The listing builds one solid part. Answer for the finished solid, in the listing's coordinates (mm). A direction names the side the tool comes from. Round coordinates to 2 decimals unless told otherwise and drop trailing zeros. One line per item, written item: value. Start each with the question number.
(1) For a pull along Y with two mould halves and no side action, classify faces 3 (the flat face through (8, 1, 0)), 4 (the flat face through (-3.12, 5.5, 8.59)), 5 (the cylindrical face through (-4.88, 37.18, 26.75)) as released by +Y, released by -Y, zero draft, split by the parting line, or undercut.
(2) Consider probe 1 along Y at (x, z) = (0, 1); probe 2 along Z at (x, y) = (13, -11); probe 3 along Y at (x, z) = (5, 10.25). Determine where each line is inside the solid, lowest interval first.
(3) For faces 1 (the flat face through (3.21, 5.45, 8.59)), 2 (the cylindrical face through (-4.88, 37.18, 0.25)), determine the directions among +Z, -Z, +X, -X, +Y, -Y from which every point of the face is accessible in a straight line to the end or side of a thin tool.
(4) Given P1, Ø8, axis at x = -26.5, z = 13.5, coming from the +Y side; P2, Ø2, axis at y = 1.5, z = 7.5, coming from the -X side; P3, Ø12, axis at x = -0.5, z = 13, coming from the +Y side, each flat-ended and moving along its own axis, determine where each tip first touches the part or whether it passes through.
```python
from build123d import *

# Parameters (mm, degrees)
ESQUISSE1_R             = 37.5
ESQUISSE1_R_2           = 2.15
BOSS_EXTRU_1_DEPTH      = 15
ESQUISSE2_R             = 37.5
ESQUISSE2_R_2           = 18.85
BOSS_EXTRU_2_DEPTH      = 12
ENL_V_MAT_EXTRU_9_DEPTH = 13
CHANFREIN1_SIZE         = 1


with BuildPart() as part:
    # Esquisse1 → Boss.-Extru.1 (new body)
    with BuildSketch(Plane.XY):
        Circle(ESQUISSE1_R)
        Circle(ESQUISSE1_R_2, mode=Mode.SUBTRACT)
    extrude(amount=BOSS_EXTRU_1_DEPTH)

    # Esquisse2 → Boss.-Extru.2 (add)
    with BuildSketch(Plane.XY.offset(15)):
        Circle(ESQUISSE2_R)
        Circle(ESQUISSE2_R_2, mode=Mode.SUBTRACT)
    extrude(amount=BOSS_EXTRU_2_DEPTH)

    # Esquisse9 → Enlèv. mat.-Extru.9 (cut)
    with BuildSketch(Plane.XY.offset(15)):
        Polygon((6.325, -3.651740453), (6.325, 3.651740453), (0, 7.303480905), (-6.325, 3.651740453), (-6.325, -3.651740453), (0, -7.303480905), align=None)
    extrude(amount=-ENL_V_MAT_EXTRU_9_DEPTH, mode=Mode.SUBTRACT)

    # Chanfrein1
    chanfrein1_edges = [part.edges().sort_by_distance(p)[0] for p in [
        (-18.85, 0, 27),
    ]]
    chamfer(chanfrein1_edges, length=CHANFREIN1_SIZE)

    # Esquisse10 → Enlèvement de matière-Révolution1 (revolve, cut)
    with BuildSketch(Plane(origin=(0, 0, 0), x_dir=(0, 0, -1), z_dir=(1, 0, 0)), mode=Mode.PRIVATE) as enl_vement_de_mati_re_r_volution1_sk:
        with BuildLine():
            Line((-26.5, 37.5), (-0.5, 37.5))
            Line((-0.5, 37.5), (-1.5, 35.5))
            ThreePointArc((-1.5, 35.5), (-13.5, 36.5), (-25.5, 35.5))
            Line((-25.5, 35.5), (-26.5, 37.5))
        make_face()
    revolve(enl_vement_de_mati_re_r_volution1_sk.sketch.rotate(Axis((0, 0, 0), (0, 0, 1)), 90), axis=Axis((0, 0, 0), (0, 0, 1)), mode=Mode.SUBTRACT)


solid = part.part
```
Recorded:
1. face 3: zero draft
1. face 4: undercut
1. face 5: split by the parting line
2. probe 1: y = -36.5 to -2.15, 2.15 to 36.5
2. probe 2: z = 0 to 15
2. probe 3: y = -36.08 to -4.42, 4.42 to 36.08
3. face 1: +Z
3. face 2: +Z, -Z
4. P1: stops at y = 28.74
4. P2: stops at x = -36.3
4. P3: stops at y = 36.5
